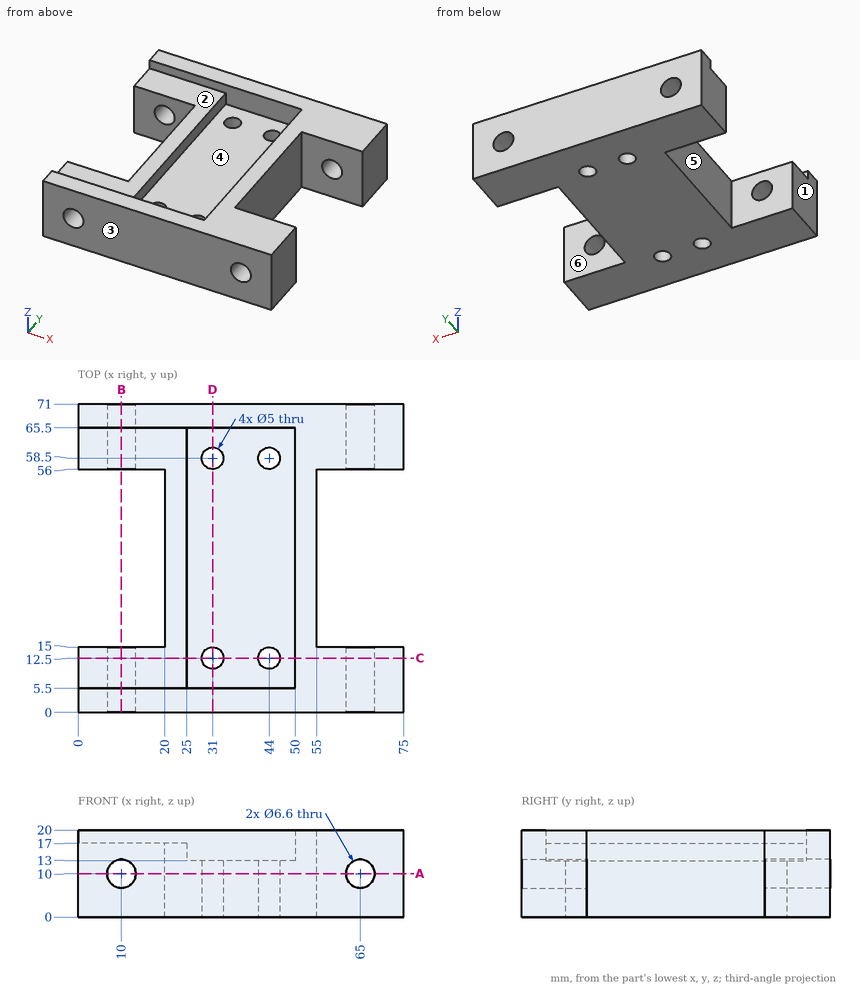
Answer from the drawing. Dimensions are ordinates in mm from the lowest x, y and z of the part. A direction names the side the tool comes from. Round coordinates to 2 decimals unless told otherwise and drop trailing zeros. Order: outer loops, then holes, each group sorted by start corner. A loop starts at its lowest first (then second) coordinate and runs counter-clockwise, first axis right, second up.
1) The part is cut by section A-A on z = 10. Give the number of separate pieces and of enclosed holes in the cut face, plus the area to 3 significant figures.
2) For the marked faces 4, 5 and 6, determine the directions among +Z, -Z, +X, -X, +Y, -Y from which every point of the face is accessible in a straight line to the end or side of a thin tool.
3) Flat-ended cylindrical pins translate along their axes: pin 1 (10 mm diameter, centred on x = 19, y = 57, fed in from +Z); pin 2 (3 mm diameter, centred on y = 31, z = 15, fed in from +X); pin 3 (8.5 mm diameter, centred on y = 37.5, z = 11, fed in from -X); pin 4 (6 mm diameter, centred on x = 16.5, z = 8, fed in from -Y). Find the tip coordinate at first contact, or state that the pin passes through.
4) The part is cut by section C-C on y = 12.5. Write down the section's boundary in (x, z), plus the area to 3 significant figures.
5) Straight lines are drawn through the part: L1, parallel to Y at x = 44, z = 7.75; L2, parallel to Y at x = 14, z = 9.5; L3, parallel to Z at x = 10, y = 6. For each, find the intervals that lie inside material, in ascending order.
6) The part is cut by section B-B on x = 10. Write down the section's boundary in (y, z).
7) The mould has two halves that part along Y. Classify the marked faces 1, 2 and 3: released by +Y, released by -Y, zero draft, split by the parting line, or undercut.
8) The part is cut by section D-D on x = 31. Write down the section's boundary in (y, z).
Resolved:
1. separate pieces: 5
1. enclosed holes: 4
1. area: 3,210 mm2
2. face 4: +Z
2. face 5: +Z, -Z, -X
2. face 6: +Z, -Z, +X
3. pin 1: stops at z = 17
3. pin 2: stops at x = 55
3. pin 3: stops at x = 20
3. pin 4: stops at y = 0
4. outline: (0, 0) - (28.5, 0) - (28.5, 13) - (25, 13) - (25, 17) - (0, 17) - close; (33.5, 0) - (41.5, 0) - (41.5, 13) - (33.5, 13) - close; (46.5, 0) - (75, 0) - (75, 20) - (50, 20) - (50, 13) - (46.5, 13) - close; hole circle Ø6.6 at (10, 10); hole circle Ø6.6 at (65, 10)
4. area: 1,050 mm2
5. L1: y = 0 to 10, 15 to 56, 61 to 71
5. L2: y = 0 to 15, 56 to 71
5. L3: z = 0 to 6.7, 13.3 to 17
6. outline: (0, 0) - (15, 0) - (15, 6.7) - (0, 6.7) - close; (0, 13.3) - (15, 13.3) - (15, 17) - (5.5, 17) - (5.5, 20) - (0, 20) - close; (56, 0) - (71, 0) - (71, 6.7) - (56, 6.7) - close; (56, 13.3) - (71, 13.3) - (71, 20) - (65.5, 20) - (65.5, 17) - (56, 17) - close
7. face 1: zero draft
7. face 2: undercut
7. face 3: released by -Y
8. outline: (0, 0) - (10, 0) - (10, 13) - (5.5, 13) - (5.5, 20) - (0, 20) - close; (15, 0) - (56, 0) - (56, 13) - (15, 13) - close; (61, 0) - (71, 0) - (71, 20) - (65.5, 20) - (65.5, 13) - (61, 13) - close
